```python
from build123d import *
from OCP.BRepFilletAPI import BRepFilletAPI_MakeChamfer

# Parameters (mm, degrees)
SKETCH1_W                                            = 239
SKETCH1_H                                            = 370
BOSS_EXTRUDE1_DEPTH                                  = 5
CSK_FOR_M3_HEX_SOCKET_COUNTERSUNK_CAP_SC_D           = 3.4
CSK_FOR_M3_HEX_SOCKET_COUNTERSUNK_CAP_SC_CSINK_D     = 6.72
CSK_FOR_M3_HEX_SOCKET_COUNTERSUNK_CAP_SC_CSINK_ANGLE = 90
SKETCH12_W                                           = 239
SKETCH12_H                                           = 3
CUT_EXTRUDE7_DEPTH                                   = 2.5
CUT_EXTRUDE8_DEPTH                                   = 441.506526626
CHAMFER1_SIZE                                        = 15
CHAMFER1_SIZE2                                       = 10.688218108
FILLET1_R                                            = 5
SKETCH14_W                                           = 209
SKETCH14_H                                           = 340
CUT_EXTRUDE9_DEPTH                                   = 2
FILLET2_R                                            = 5
M3_TAPPED_HOLE1_D                                    = 2.5
M3_TAPPED_HOLE1_DEPTH                                = 15
M3_TAPPED_HOLE1_TIP                                  = 0.751075774


with BuildPart() as part:
    # Sketch1 → Boss-Extrude1 (new body)
    with BuildSketch(Plane(origin=(0, 0, 0), x_dir=(1, 0, 0), z_dir=(0, 1, 0))):
        with Locations((-119.5, 185)):
            Rectangle(SKETCH1_W, SKETCH1_H)
    extrude(amount=BOSS_EXTRUDE1_DEPTH)

    # CSK for M3 Hex Socket Countersunk Cap Screw1 (through all)
    with Locations(Plane(origin=(0, 5, 0), x_dir=(1, 0, 0), z_dir=(0, 1, 0))):
        with Locations((-3.5, 15), (-3.5, 100), (-3.5, 185), (-3.5, 270), (-3.5, 355)):
            csk_for_m3_hex_socket_countersunk_cap_sc = CounterSinkHole(CSK_FOR_M3_HEX_SOCKET_COUNTERSUNK_CAP_SC_D / 2, CSK_FOR_M3_HEX_SOCKET_COUNTERSUNK_CAP_SC_CSINK_D / 2, counter_sink_angle=CSK_FOR_M3_HEX_SOCKET_COUNTERSUNK_CAP_SC_CSINK_ANGLE)

    # Mirror1: CSK for M3 Hex Socket Countersunk Cap Screw1 across plane
    add(csk_for_m3_hex_socket_countersunk_cap_sc.mirror(Plane.ZY.offset(119.5)), mode=Mode.SUBTRACT)

    # Sketch12 → Cut-Extrude7 (cut)
    with BuildSketch(Plane.XZ):
        with Locations((-119.5, -1.5)):
            Rectangle(SKETCH12_W, SKETCH12_H)
        with Locations((-119.5, -368.5)):
            Rectangle(SKETCH12_W, SKETCH12_H)
    extrude(amount=-CUT_EXTRUDE7_DEPTH, mode=Mode.SUBTRACT)

    # Sketch13 → Cut-Extrude8 (cut, through all)
    with BuildSketch(Plane(origin=(0, 5, 0), x_dir=(1, 0, 0), z_dir=(0, 1, 0))):
        Polygon((-20, 39.013212111), (-20, 175), (-194.589488967, 175), align=None)
        Polygon((-20, 350), (-219, 350), (-219, 195), align=None)
        Polygon((-20, 330.986787889), (-20, 195), (-194.589488967, 195), align=None)
        Polygon((-219, 20), (-219, 175), (-20, 20), align=None)
    extrude(amount=-CUT_EXTRUDE8_DEPTH, mode=Mode.SUBTRACT)

    # Chamfer1: one chamfer whose edges measure the first distance from different faces: ONE call of the kernel's chamfer builder (chamfer() names one face for all edges)
    chamfer1_edges_1 = [part.edges().sort_by_distance(p)[0] for p in [
        (-20, 2.5, -20),
    ]]
    chamfer1_side_1 = [part.faces().sort_by_distance(p)[0] for p in [
        (-119.5, 2.5, -20),
    ]]
    chamfer1_edges_2 = [part.edges().sort_by_distance(p)[0] for p in [
        (-219, 2.5, -20),
        (-20, 2.5, -175),
        (-219, 2.5, -350),
        (-20, 2.5, -195),
    ]]
    chamfer1_edges_3 = [part.edges().sort_by_distance(p)[0] for p in [
        (-219, 2.5, -175),
    ]]
    chamfer1_side_3 = [part.faces().sort_by_distance(p)[0] for p in [
        (-119.5, 2.5, -97.5),
    ]]
    chamfer1_edges_4 = [part.edges().sort_by_distance(p)[0] for p in [
        (-194.589488967, 2.5, -175),
    ]]
    chamfer1_side_4 = [part.faces().sort_by_distance(p)[0] for p in [
        (-107.294744483, 2.5, -175),
    ]]
    chamfer1_edges_5 = [part.edges().sort_by_distance(p)[0] for p in [
        (-20, 2.5, -39.013212111),
    ]]
    chamfer1_side_5 = [part.faces().sort_by_distance(p)[0] for p in [
        (-107.294744483, 2.5, -107.006606056),
    ]]
    chamfer1_edges_6 = [part.edges().sort_by_distance(p)[0] for p in [
        (-20, 2.5, -350),
    ]]
    chamfer1_side_6 = [part.faces().sort_by_distance(p)[0] for p in [
        (-119.5, 2.5, -272.5),
    ]]
    chamfer1_edges_7 = [part.edges().sort_by_distance(p)[0] for p in [
        (-219, 2.5, -195),
    ]]
    chamfer1_side_7 = [part.faces().sort_by_distance(p)[0] for p in [
        (-219, 2.5, -272.5),
    ]]
    chamfer1_edges_8 = [part.edges().sort_by_distance(p)[0] for p in [
        (-194.589488967, 2.5, -195),
    ]]
    chamfer1_side_8 = [part.faces().sort_by_distance(p)[0] for p in [
        (-107.294744483, 2.5, -262.993393944),
    ]]
    chamfer1_edges_9 = [part.edges().sort_by_distance(p)[0] for p in [
        (-20, 2.5, -330.986787889),
    ]]
    chamfer1_side_9 = [part.faces().sort_by_distance(p)[0] for p in [
        (-20, 2.5, -262.993393944),
    ]]
    chamfer1 = BRepFilletAPI_MakeChamfer(part.part.solid().wrapped)
    for e in chamfer1_edges_1:
        chamfer1.Add(CHAMFER1_SIZE, CHAMFER1_SIZE2, e.wrapped, chamfer1_side_1[0].wrapped)  # the first distance lies on this face
    for e in chamfer1_edges_2:
        chamfer1.Add(CHAMFER1_SIZE, e.wrapped)
    for e in chamfer1_edges_3:
        chamfer1.Add(CHAMFER1_SIZE, CHAMFER1_SIZE2, e.wrapped, chamfer1_side_3[0].wrapped)  # the first distance lies on this face
    for e in chamfer1_edges_4:
        chamfer1.Add(CHAMFER1_SIZE, CHAMFER1_SIZE2, e.wrapped, chamfer1_side_4[0].wrapped)  # the first distance lies on this face
    for e in chamfer1_edges_5:
        chamfer1.Add(CHAMFER1_SIZE, CHAMFER1_SIZE2, e.wrapped, chamfer1_side_5[0].wrapped)  # the first distance lies on this face
    for e in chamfer1_edges_6:
        chamfer1.Add(CHAMFER1_SIZE, CHAMFER1_SIZE2, e.wrapped, chamfer1_side_6[0].wrapped)  # the first distance lies on this face
    for e in chamfer1_edges_7:
        chamfer1.Add(CHAMFER1_SIZE, CHAMFER1_SIZE2, e.wrapped, chamfer1_side_7[0].wrapped)  # the first distance lies on this face
    for e in chamfer1_edges_8:
        chamfer1.Add(CHAMFER1_SIZE, CHAMFER1_SIZE2, e.wrapped, chamfer1_side_8[0].wrapped)  # the first distance lies on this face
    for e in chamfer1_edges_9:
        chamfer1.Add(CHAMFER1_SIZE, CHAMFER1_SIZE2, e.wrapped, chamfer1_side_9[0].wrapped)  # the first distance lies on this face
    add(Compound.cast(chamfer1.Shape()), mode=Mode.REPLACE)

    # Fillet1
    fillet1_edges = [part.edges().sort_by_distance(p)[0] for p in [
        (-179.589488967, 2.5, -175),
        (-35, 2.5, -175),
        (-20, 2.5, -49.701430219),
        (-20, 2.5, -160),
        (-219, 2.5, -35),
        (-219, 2.5, -164.311781892),
        (-28.43220339, 2.5, -26.56779661),
        (-207.16612371, 2.5, -165.782659171),
        (-204, 2.5, -20),
        (-35, 2.5, -20),
        (-186.157285577, 2.5, -168.43220339),
        (-31.83387629, 2.5, -48.23055294),
        (-31.83387629, 2.5, -340.782659171),
        (-210.56779661, 2.5, -201.56779661),
        (-219, 2.5, -335),
        (-219, 2.5, -210),
        (-35, 2.5, -195),
        (-183.901270859, 2.5, -195),
        (-28.43220339, 2.5, -324.418991278),
        (-182.755612677, 2.5, -204.217340829),
        (-20, 2.5, -210),
        (-20, 2.5, -315.986787889),
        (-204, 2.5, -350),
        (-30.688218108, 2.5, -350),
    ]]
    fillet(fillet1_edges, radius=FILLET1_R)

    # Sketch14 → Cut-Extrude9 (cut)
    with BuildSketch(Plane(origin=(0, 5, 0), x_dir=(1, 0, 0), z_dir=(0, 1, 0))):
        with Locations((-119.5, 185)):
            Rectangle(SKETCH14_W, SKETCH14_H)
    extrude(amount=-CUT_EXTRUDE9_DEPTH, mode=Mode.SUBTRACT)

    # Fillet2
    fillet2_edges = [part.edges().sort_by_distance(p)[0] for p in [
        (-224, 4, -15),
        (-224, 4, -355),
        (-15, 4, -355),
        (-15, 4, -15),
    ]]
    fillet(fillet2_edges, radius=FILLET2_R)

    # M3 Tapped Hole1
    with Locations(Plane(origin=(0, 3, 0), x_dir=(1, 0, 0), z_dir=(0, 1, 0))):
        with Locations((-219, 350), (-20, 350), (-20, 20), (-27.5, 192.5), (-219, 20), (-27.5, 177.5), (-199, 195.577889447), (-199, 174.422110553)):
            Hole(M3_TAPPED_HOLE1_D / 2, depth=M3_TAPPED_HOLE1_DEPTH)
            with Locations((0, 0, -(M3_TAPPED_HOLE1_DEPTH + M3_TAPPED_HOLE1_TIP / 2))):  # 118° drill point
                Cone(0, M3_TAPPED_HOLE1_D / 2, M3_TAPPED_HOLE1_TIP, mode=Mode.SUBTRACT)


solid = part.part
```
Input: part model. Units: mm. Frame: model coordinates. A direction names the side the tool comes from. Give positions to 0.01 mm unless a question says otherwise; leave off trailing zeros. Order: outer loops, then holes, each group sorted by start corner. A loop starts at its lowest first (then second) coordinate and runs counter-clockwise, first axis right, second up.
1. Section B-B on x = -143.5. Return the cut outline in (y, z), and give its area (3 significant figures).
Derived:
outline: (0, -367) - (2.5, -367) - (2.5, -370) - (5, -370) - (5, -355) - (3, -355) - (3, -350) - (0, -350) - close; (0, -253.81) - (3, -253.81) - (3, -234.79) - (0, -234.79) - close; (0, -195) - (3, -195) - (3, -175) - (0, -175) - close; (0, -135.21) - (3, -135.21) - (3, -116.19) - (0, -116.19) - close; (0, -20) - (3, -20) - (3, -15) - (5, -15) - (5, 0) - (2.5, 0) - (2.5, -3) - (0, -3) - close
area: 339 mm2
2. Pin query (flat end, axial travel): pin 1 (3 mm diameter, centred on x = -235.5, z = -15, fed in from -Y); pin 2 (0.9 mm diameter, centred on x = -88, y = 2, fed in from +Z); pin 3 (2 mm diameter, centred on x = -160.5, y = 4, fed in from +Z); pin 4 (2.5 mm diameter, centred on x = -114, y = 1, fed in from -Z). Return the tip coordinate at first contact, or that it passes through.
Derived:
pin 1: passes through
pin 2: stops at z = -3
pin 3: stops at z = 0
pin 4: stops at z = -367
3. Mould query, pull axis Z, two halves, no side actions, for faces 4 (the flat face through (-121, 0, -188)), 5 (the flat face through (-120.4, 1.5, -98.2)). Classes: released by +Z, released by -Z, zero draft, split by the parting line, or undercut.
Derived:
face 4: zero draft
face 5: undercut
4. Section C-C on y = 1.1. Give the number of separate pieces and of enclosed holes in the cut face, and give its area (3 significant figures).
Derived:
separate pieces: 1
enclosed holes: 22
area: 33,200 mm2
5. Reachability of faces 1 (the flat face through (-120, 3, -186)), 2 (the flat face through (-226, 5, -186)), 3 (the flat face through (-212, 2, -28)) from +Z, -Z, +X, -X, +Y, -Y: full face, straight path, thin tool, end or side. Return the list, or none.
Derived:
face 1: +Y
face 2: +Z, -Z, +X, -X, +Y
face 3: +Y, -Y
6. Material intervals for L1, parallel to Z at x = -235.5, y = 1.75; L2, parallel to X at y = 0.9, z = -185; L3, parallel to X at y = 3.35, z = -321.5, sorted ascending.
Derived:
L1: z = -367 to -356.7, -353.3 to -271.7, -268.3 to -186.7, -183.3 to -101.7, -98.3 to -16.7, -13.3 to -3
L2: x = -239 to -237.2, -233.8 to -5.2, -1.8 to 0
L3: x = -239 to -224, -15 to 0
7. Section A-A on z = -142. Return the cut outline in (x, y), and give its area (3 significant figures).
Derived:
outline: (-239, 0) - (-219, 0) - (-219, 3) - (-224, 3) - (-224, 5) - (-239, 5) - close; (-176.63, 0) - (-152.22, 0) - (-152.22, 3) - (-176.63, 3) - close; (-20, 0) - (0, 0) - (0, 5) - (-15, 5) - (-15, 3) - (-20, 3) - close
area: 253 mm2
